CAD build for the part. Positions are in the model's coordinates, mm. Face numbers are marked on the shaded views. A direction names the side the tool comes from. Give positions to 0.01 mm unless a question says otherwise; leave off trailing zeros. Write each loop counter-clockwise with the first axis right and the second up, starting at its lowest first coordinate (ties: lowest second). Pieces come first, ordered by that corner, then holes. Notation, with made-up numbers: (88, 79.5) -> (134, 79.5) arc R23 ccw to (134, 106.5) -> close; hole circle Ø9 at (67, 5.5). An arc over 180 degrees is marked (long way). Answer in a Markdown table with one row per item. Add a question column.
```python
from build123d import *

# Parameters (mm, degrees)
SKETCH1_R           = 2.2479
BOSS_EXTRUDE1_DEPTH = 2.54
FILLET1_R           = 5.08
SKETCH2_W           = 38.1
SKETCH2_H           = 38.1
SKETCH2_R           = 2.54
BOSS_EXTRUDE2_DEPTH = 2.54
FILLET2_R           = 2.54
FILLET3_R           = 2.54


with BuildPart() as part:
    # Sketch1 → Boss-Extrude1 (new body)
    with BuildSketch(Plane(origin=(0, 0, 0), x_dir=(1, 0, 0), z_dir=(0, 1, 0))):
        Polygon((-19.583364039, 16.770768135), (-5.08, 16.770768135), (-5.08, -1.009231865), (5.08, -1.009231865), (5.08, 16.770768135), (18.516635961, 16.770768135), (18.516635961, -14.979231865), (-19.583364039, -14.979231865), align=None)
        with Locations(Location((-12.839664039, 4.070768135, 0), (0, 0, 270))):
            Circle(SKETCH1_R, mode=Mode.SUBTRACT)
        with Locations(Location((11.772935961, 4.070768135, 0), (0, 0, 270))):
            Circle(SKETCH1_R, mode=Mode.SUBTRACT)
    extrude(amount=BOSS_EXTRUDE1_DEPTH)

    # Fillet1
    fillet1_edges = [part.edges().sort_by_distance(p)[0] for p in [
        (5.08, 1.27, 1.009231865),
        (-5.08, 1.27, 1.009231865),
    ]]
    fillet(fillet1_edges, radius=FILLET1_R - 0.0001)  # a hair under: the kernel refuses the full size

    # Sketch2 → Boss-Extrude2 (add)
    with BuildSketch(Plane.XY.offset(14.979231865)):
        with Locations((-0.533364039, -16.51)):
            Rectangle(SKETCH2_W, SKETCH2_H)
        with Locations((-0.533364039, -12.7)):
            Circle(SKETCH2_R, mode=Mode.SUBTRACT)
        with Locations((-0.533364039, -26.67)):
            Circle(SKETCH2_R, mode=Mode.SUBTRACT)
    extrude(amount=BOSS_EXTRUDE2_DEPTH)

    # Fillet2
    fillet2_edges = [part.edges().sort_by_distance(p)[0] for p in [
        (-0.533364039, 0, 14.979231865),
    ]]
    fillet(fillet2_edges, radius=FILLET2_R)

    # Fillet3
    fillet3_edges = [part.edges().sort_by_distance(p)[0] for p in [
        (-0.533364039, 2.54, 17.519231865),
    ]]
    fillet(fillet3_edges, radius=FILLET3_R)


solid = part.part
```
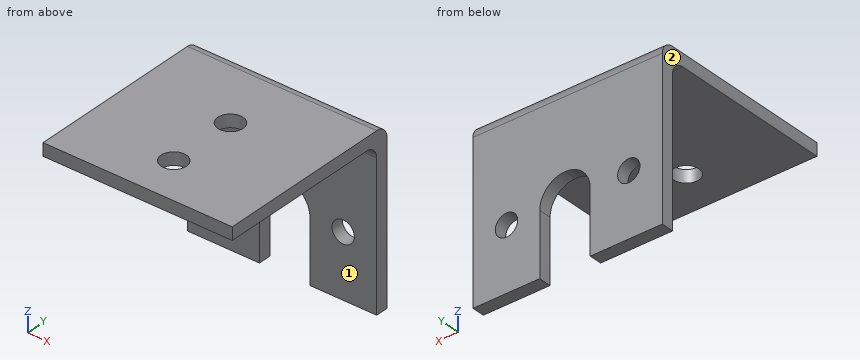
Item 1: Which spindle directions (+Z, -Z, +X, -X, +Y, -Y) get a long thin tool onto all of the face, cutting with end or side? Do the marked faces 1 and 2. Say none if no direction does.
Item 2: Slice it at D-D, the plane y = -17. List the corners of the cut face in (x, z), then the cut area to 3 significant figures.
Item 3: Slice it at C-C, the plane x = 13. List the corners of the cut face in (y, z), then the cut area to 3 significant figures.
Item 4: Probe L1, parallel to Z at x = 12.5, y = -22.5; L2, parallel to Y at x = 8.5, z = 10; L3, parallel to X at y = -12, z = 16 (3 decimals). List the from-to ranges inside material, lowest first. Write a range as from..to.
Item 5: Drop flat-ended pins along their axis: pin 1 Ø10 at (x, z) = (-5, -4.5) entering from -Y; pin 2 Ø4.5 at (x, y) = (-0.53, -26.67) entering from +Z; pin 3 Ø10 at (x, z) = (-4.5, -11.5) entering from +Y; pin 4 Ø6 at (x, y) = (-0.53, -12.7) entering from -Z. Give the stop position or say it passes through.
Item 6: Slice it at B-B, the plane y = -12.7. List the corners of the cut face in (x, z), then the cut area to 3 significant figures.
Item 7: Slice it at A-A, the plane z = -12. List the corners of the cut face in (x, y), then the cut area to 3 significant figures.
Answer key:
| question | item | result |
|---|---|---|
| 1 | face 1 | -Z, +X, -X, -Y |
| 1 | face 2 | +Z, -Z, -X, +Y, -Y |
| 2 | outline | (-19.58, 14.98) -> (18.52, 14.98) -> (18.52, 17.52) -> (-19.58, 17.52) -> close |
| 2 | area | 96.8 mm² |
| 3 | outline | (-35.56, 14.98) -> (-2.54, 14.98) arc R2.54 cw to (0, 12.44) -> (0, -2.19) -> (2.54, -2.19) -> (2.54, 14.98) arc R2.54 ccw to (0, 17.52) -> (-35.56, 17.52) -> close; (0, -16.77) -> (2.54, -16.77) -> (2.54, -5.95) -> (0, -5.95) -> close |
| 3 | area | 168 mm² |
| 4 | L1 | z = 14.98..17.52 |
| 4 | L2 | y = 0..2.54 |
| 4 | L3 | x = -19.583..-2.975, 1.908..18.517 |
| 5 | pin 1 | stops at y = 0 |
| 5 | pin 2 | passes through |
| 5 | pin 3 | stops at y = 2.54 |
| 5 | pin 4 | stops at z = 14.98 |
| 6 | outline | (-19.58, 14.98) -> (-3.07, 14.98) -> (-3.07, 17.52) -> (-19.58, 17.52) -> close; (2.01, 14.98) -> (18.52, 14.98) -> (18.52, 17.52) -> (2.01, 17.52) -> close |
| 6 | area | 83.9 mm² |
| 7 | outline | (-19.58, 0) -> (-5.08, 0) -> (-5.08, 2.54) -> (-19.58, 2.54) -> close; (5.08, 0) -> (18.52, 0) -> (18.52, 2.54) -> (5.08, 2.54) -> close |
| 7 | area | 71.0 mm² |
